from build123d import *

# Parameters (mm, degrees)
ESQUISSE1_R                                   = 3
ESQUISSE1_R_2                                 = 10.1
ESQUISSE1_R_3                                 = 1.5
ESQUISSE1_W                                   = 25
ESQUISSE1_H                                   = 60
ESQUISSE1_W_2                                 = 20
ESQUISSE1_H_2                                 = 30
BOSS_EXTRU_1_DEPTH                            = 5
CONG_1_R                                      = 3
ESQUISSE3_R                                   = 4.2
ENL_V_MAT_EXTRU_2_DEPTH                       = 4
ESQUISSE4_W                                   = 9
ESQUISSE4_H                                   = 56
ENL_V_MAT_EXTRU_3_DEPTH                       = 2
TROU_POUR_TARAUDAGE_POUR_TROU_TARAUD_M4_D     = 3.3
TROU_POUR_TARAUDAGE_POUR_TROU_TARAUD_M4_DEPTH = 10
TROU_POUR_TARAUDAGE_POUR_TROU_TARAUD_M4_TIP   = 0.991420021


with BuildPart() as part:
    # Esquisse1 → Boss.-Extru.1 (new body)
    with BuildSketch(Plane(origin=(0, 0, 0), x_dir=(1, 0, 0), z_dir=(0, 1, 0))):
        Polygon((-104, 95), (-104, -95), (-80, -105), (-51, -105), (-51, -40), (-9, -40), (-9, -25), (0, -25), (0, 25), (-9, 25), (-9, 40), (-51, 40), (-51, 105), (-80, 105), align=None)
        with Locations(Location((-60, 30, 0), (0, 0, 270))):
            Circle(ESQUISSE1_R, mode=Mode.SUBTRACT)
        with Locations(Location((-60, -30, 0), (0, 0, 270))):
            Circle(ESQUISSE1_R, mode=Mode.SUBTRACT)
        with Locations(Location((-19, -30, 0), (0, 0, 270))):
            Circle(ESQUISSE1_R, mode=Mode.SUBTRACT)
        with Locations(Location((-19, 30, 0), (0, 0, 270))):
            Circle(ESQUISSE1_R, mode=Mode.SUBTRACT)
        with Locations(Location((-94, 85, 0), (0, 0, 270))):
            Circle(ESQUISSE1_R, mode=Mode.SUBTRACT)
        with Locations(Location((-94, -85, 0), (0, 0, 270))):
            Circle(ESQUISSE1_R, mode=Mode.SUBTRACT)
        with Locations(Location((-66.7, 89.3, 0), (0, 0, 270))):
            Circle(ESQUISSE1_R_2, mode=Mode.SUBTRACT)
        with Locations(Location((-54, 89.3, 0), (0, 0, 270))):
            Circle(ESQUISSE1_R_3, mode=Mode.SUBTRACT)
        with Locations(Location((-66.7, 102, 0), (0, 0, 270))):
            Circle(ESQUISSE1_R_3, mode=Mode.SUBTRACT)
        with Locations(Location((-79.4, 89.3, 0), (0, 0, 270))):
            Circle(ESQUISSE1_R_3, mode=Mode.SUBTRACT)
        with Locations(Location((-66.7, 76.6, 0), (0, 0, 270))):
            Circle(ESQUISSE1_R_3, mode=Mode.SUBTRACT)
        with Locations(Location((-66.7, -89.3, 0), (0, 0, 270))):
            Circle(ESQUISSE1_R_2, mode=Mode.SUBTRACT)
        with Locations(Location((-54, -89.3, 0), (0, 0, 270))):
            Circle(ESQUISSE1_R_3, mode=Mode.SUBTRACT)
        with Locations(Location((-66.7, -76.6, 0), (0, 0, 270))):
            Circle(ESQUISSE1_R_3, mode=Mode.SUBTRACT)
        with Locations(Location((-79.4, -89.3, 0), (0, 0, 270))):
            Circle(ESQUISSE1_R_3, mode=Mode.SUBTRACT)
        with Locations(Location((-66.7, -102, 0), (0, 0, 270))):
            Circle(ESQUISSE1_R_3, mode=Mode.SUBTRACT)
        with Locations((-36.5, 0)):
            Rectangle(ESQUISSE1_W, ESQUISSE1_H, mode=Mode.SUBTRACT)
        with BuildLine():
            Line((-88, 22), (-88, -22))
            ThreePointArc((-88, -22), (-92, -26), (-96, -22))
            Line((-96, -22), (-96, 22))
            ThreePointArc((-96, 22), (-92, 26), (-88, 22))
        make_face(mode=Mode.SUBTRACT)
        with Locations((-74, 0)):
            Rectangle(ESQUISSE1_W_2, ESQUISSE1_H_2, mode=Mode.SUBTRACT)
    extrude(amount=BOSS_EXTRU_1_DEPTH)

    # Congé1
    cong_1_edges = [part.edges().sort_by_distance(p)[0] for p in [
        (-51, 2.5, -105),
        (-51, 2.5, -40),
        (-9, 2.5, -40),
        (-9, 2.5, -25),
        (0, 2.5, -25),
        (0, 2.5, 25),
        (-9, 2.5, 25),
        (-9, 2.5, 40),
        (-51, 2.5, 40),
        (-51, 2.5, 105),
        (-49, 2.5, -30),
        (-49, 2.5, 30),
        (-24, 2.5, 30),
        (-24, 2.5, -30),
        (-84, 2.5, -15),
        (-84, 2.5, 15),
        (-64, 2.5, 15),
        (-64, 2.5, -15),
    ]]
    fillet(cong_1_edges, radius=CONG_1_R)

    # Esquisse3 → Enlèv. mat.-Extru.2 (cut)
    with BuildSketch(Plane(origin=(0, 5, 0), x_dir=(1, 0, 0), z_dir=(0, 1, 0))):
        with Locations(Location((-93, 40.65, 0), (0, 0, 270))):
            Circle(ESQUISSE3_R)
        with Locations(Location((-93, -40.45, 0), (0, 0, 270))):
            Circle(ESQUISSE3_R)
    extrude(amount=-ENL_V_MAT_EXTRU_2_DEPTH, mode=Mode.SUBTRACT)

    # Esquisse4 → Enlèv. mat.-Extru.3 (cut)
    with BuildSketch(Plane(origin=(0, 5, 0), x_dir=(1, 0, 0), z_dir=(0, 1, 0))):
        with Locations((-4.5, 0)):
            Rectangle(ESQUISSE4_W, ESQUISSE4_H)
    extrude(amount=-ENL_V_MAT_EXTRU_3_DEPTH, mode=Mode.SUBTRACT)

    # Trou pour taraudage pour trou taraudé M41
    with Locations(Plane(origin=(0, 3, 0), x_dir=(1, 0, 0), z_dir=(0, 1, 0))):
        with Locations((-4, 15), (-4, -15)):
            Hole(TROU_POUR_TARAUDAGE_POUR_TROU_TARAUD_M4_D / 2, depth=TROU_POUR_TARAUDAGE_POUR_TROU_TARAUD_M4_DEPTH)
            with Locations((0, 0, -(TROU_POUR_TARAUDAGE_POUR_TROU_TARAUD_M4_DEPTH + TROU_POUR_TARAUDAGE_POUR_TROU_TARAUD_M4_TIP / 2))):  # 118° drill point
                Cone(0, TROU_POUR_TARAUDAGE_POUR_TROU_TARAUD_M4_D / 2, TROU_POUR_TARAUDAGE_POUR_TROU_TARAUD_M4_TIP, mode=Mode.SUBTRACT)


solid = part.part
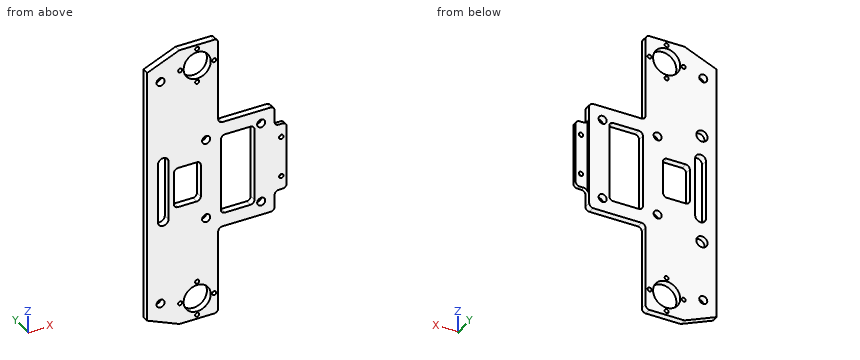
The model under review builds one solid part; all positions refer to its coordinate system, in mm. Coordinates: 2 decimals unless noted, no trailing zeros. Write each loop counter-clockwise with the first axis right and the second up, starting at its lowest first coordinate (ties: lowest second). Pieces come first, ordered by that corner, then holes. Notation, with made-up numbers: M 83,25 L 111,25 A19 cw 111,60 Z; hole C -39.5,72.5 d5. An arc over 180 degrees is marked long. Put each result on its own line as item: value.
1) Add section D-D on x = -86. Give the boundary of the cut face in (y, z).
Computed:
outline: M 0,-102.5 L 5,-102.5 L 5,102.5 L 0,102.5 Z
2) Clearance check with flat-ended pins moving along their axes: pin 1 Ø3 at (y, z) = (1, 23) entering from +X; pin 2 Ø4.5 at (x, z) = (-4, -15) entering from +Y; pin 3 Ø2 at (y, z) = (1.5, 51.5) entering from +X. State where each tip first meets the part, or that it passes through.
Computed:
pin 1: stops at x = 0
pin 2: stops at y = 3
pin 3: stops at x = -51
3) Wall thickness on probe 1 along X at (y, z) = (4.3, 4); probe 2 along X at (y, z) = (3.55, -89.3); probe 3 along Z at (x, y) = (-33, 3.2): over which ranges is each line inside the solid? List them lowest first. Write a range as [from, to].
Computed:
probe 1: x = [-104, -96], [-88, -84], [-64, -49], [-24, -9]
probe 2: x = [-104, -80.9], [-77.9, -76.8], [-56.6, -55.5], [-52.5, -51]
probe 3: z = [-40, -30], [30, 40]
4) Add section C-C on z = -85. Give the boundary of the cut face in (x, y), then the cut area to 3 significant figures.
Computed:
outline: M -104,0 L -97,0 L -97,5 L -104,5 Z; M -91,0 L -75.84,0 L -75.84,5 L -91,5 Z; M -57.56,0 L -51,0 L -51,5 L -57.56,5 Z
area: 144 mm2
5) Add section A-A on z = 8. Give the boundary of the cut face in (x, y), then the cut area to 3 significant figures.
Computed:
outline: M -104,0 L -96,0 L -96,5 L -104,5 Z; M -88,0 L -84,0 L -84,5 L -88,5 Z; M -64,0 L -49,0 L -49,5 L -64,5 Z; M -24,0 L 0,0 L 0,3 L -9,3 L -9,5 L -24,5 Z
area: 237 mm2
6) Add section B-B on x = -60. Give the boundary of the cut face in (y, z), then the cut area to 3 significant figures.
Computed:
outline: M 0,-105 L 5,-105 L 5,-96.86 L 0,-96.86 Z; M 0,-81.74 L 5,-81.74 L 5,-33 L 0,-33 Z; M 0,-27 L 5,-27 L 5,27 L 0,27 Z; M 0,33 L 5,33 L 5,81.74 L 0,81.74 Z; M 0,96.86 L 5,96.86 L 5,105 L 0,105 Z
area: 839 mm2
